Model file for the job. Use its own axes, mm. Face numbers are marked on the shaded views. A direction names the side the tool comes from. Coordinates: 2 decimals unless noted, no trailing zeros. Loops run counter-clockwise (first coordinate to the right, second up) from the corner with the lowest first, then second, coordinate; pieces in that order, holes last. Notation, with made-up numbers: M 6.5,7 L 44.5,7 A21 cw 44.5,35 Z; hole C 21,89.25 d6. An arc over 180 degrees is marked long. One line per question, with ' | ' between items. Start each with the question number.
```python
from build123d import *

# Parameters (mm, degrees)
SKETCH2_R               = 1
CUT_EXTRUDE1_DEPTH      = 5
CUT_EXTRUDE2_DEPTH      = 5
CUT_EXTRUDE3_DEPTH      = 68.470363864
CUT_EXTRUDE3_DEPTH_BACK = 68.470363864


with BuildPart() as part:
    # Sketch1 → Revolve1 (revolve)
    with BuildSketch(Plane(origin=(0, 0, 0), x_dir=(0, 0, -1), z_dir=(1, 0, 0)), mode=Mode.PRIVATE) as revolve1_sk:
        Polygon((0, 0), (1.15, 0), (1.15, 12), (5, 12), (5, 15), (14, 15), (14, 61.5), (5, 61.5), (5, 64.5), (0, 64.5), align=None)
    revolve(revolve1_sk.sketch.rotate(Axis((0, 64.5, 0), (0, -1, 0)), 180), axis=Axis((0, 64.5, 0), (0, -1, 0)))

    # Sketch2 → Cut-Extrude1 (cut)
    with BuildSketch(Plane.XZ.offset(-15)):
        with Locations(Location((-8, 0, 0), (0, 0, 270))):
            Circle(SKETCH2_R)
        with Locations(Location((8, 0, 0), (0, 0, 270))):
            Circle(SKETCH2_R)
    extrude(amount=-CUT_EXTRUDE1_DEPTH, mode=Mode.SUBTRACT)

    # Sketch3 → Cut-Extrude2 (cut)
    with BuildSketch(Plane.XZ.offset(-15)):
        with BuildLine():
            ThreePointArc((-5.070033124, 9.19482268), (-7.424621202, 7.424621202), (-9.19482268, 5.070033124))
            ThreePointArc((-9.19482268, 5.070033124), (-8.60556703, 3.03219658), (-6.567730486, 3.621452231))
            ThreePointArc((-6.567730486, 3.621452231), (-5.303300859, 5.303300859), (-3.621452231, 6.567730486))
            ThreePointArc((-3.621452231, 6.567730486), (-3.03219658, 8.60556703), (-5.070033124, 9.19482268))
        make_face()
        with BuildLine():
            ThreePointArc((6.567730486, 3.621452231), (5.303300859, 5.303300859), (3.621452231, 6.567730486))
            ThreePointArc((3.621452231, 6.567730486), (3.03219658, 8.60556703), (5.070033124, 9.19482268))
            ThreePointArc((5.070033124, 9.19482268), (7.424621202, 7.424621202), (9.19482268, 5.070033124))
            ThreePointArc((9.19482268, 5.070033124), (8.60556703, 3.03219658), (6.567730486, 3.621452231))
        make_face()
        with BuildLine():
            ThreePointArc((3.621452231, -6.567730486), (5.303300859, -5.303300859), (6.567730486, -3.621452231))
            ThreePointArc((6.567730486, -3.621452231), (8.60556703, -3.03219658), (9.19482268, -5.070033124))
            ThreePointArc((9.19482268, -5.070033124), (7.424621202, -7.424621202), (5.070033124, -9.19482268))
            ThreePointArc((5.070033124, -9.19482268), (3.03219658, -8.60556703), (3.621452231, -6.567730486))
        make_face()
        with BuildLine():
            ThreePointArc((-6.567730486, -3.621452231), (-5.303300859, -5.303300859), (-3.621452231, -6.567730486))
            ThreePointArc((-3.621452231, -6.567730486), (-3.03219658, -8.60556703), (-5.070033124, -9.19482268))
            ThreePointArc((-5.070033124, -9.19482268), (-7.424621202, -7.424621202), (-9.19482268, -5.070033124))
            ThreePointArc((-9.19482268, -5.070033124), (-8.60556703, -3.03219658), (-6.567730486, -3.621452231))
        make_face()
    extrude(amount=-CUT_EXTRUDE2_DEPTH, mode=Mode.SUBTRACT)

    # Sketch4 → Cut-Extrude3 (cut, two sides: drawn at the far end of the back side and taken through both)
    with BuildSketch(Plane(origin=(0, 0, 0), x_dir=(0, 0, -1), z_dir=(1, 0, 0)).offset(-CUT_EXTRUDE3_DEPTH_BACK)):
        with BuildLine():
            Line((-5, 56), (5, 56))
            ThreePointArc((5, 56), (7, 54), (5, 52))
            Line((5, 52), (-5, 52))
            ThreePointArc((-5, 52), (-7, 54), (-5, 56))
        make_face()
    extrude(amount=CUT_EXTRUDE3_DEPTH + CUT_EXTRUDE3_DEPTH_BACK, mode=Mode.SUBTRACT)


solid = part.part
```
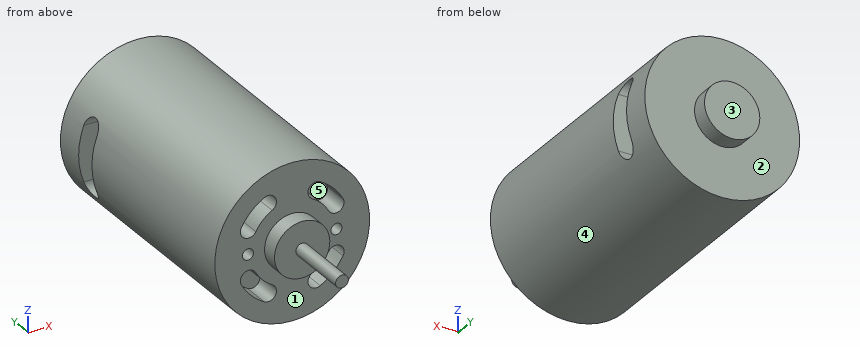
(1) Drill centre lines: line 1 (X direction, y = 17.3, z = 0); line 2 (Z direction, x = -5.5, y = 19); line 3 (Y direction, x = 7, z = -3.25). Where is each one in solid material? Low to high. Write a range as [from, to].
(2) Band-saw the part on B-B on z = 0. Write the cut outline in (x, y).
(3) Band-saw the part on A-A on x = 0. Write the cut outline in (y, z).
(4) Two-plate mould, pull along Z, no slides. Class the marked faces 3, 4 and 5: pulls with the +Z half, pulls with the -Z half, needs draft (parallel to the pull), parting line crosses it, or undercut.
(5) Band-saw the part on C-C on y = 55. Write the cut outline in (x, z).
(6) 3-axis set-ups, long thin cutter, end or side, ignore diameter. For the marked faces 1 and 2: which of +Z, -Z, +X, -X, +Y, -Y reach the whole face in a straight line?
(7) Band-saw the part on D-D on x = 10.75. Write the cut outline in (y, z), then the cut area to 3 significant figures.
(8) Pin check, flat tips, straight feed: P1, Ø1.5, axis at x = 3.5, y = 21.5, coming from the -Z side; P2, Ø3, axis at x = 3.5, z = 0, coming from the -Y side; P3, Ø5, axis at x = -6, z = -7.5, coming from the -Y side. Stop position of each tip, or through.
Computed values:
1) line 1: [-14, -9], [-7, 7], [9, 14] | line 2: [-12.87, -8.94], [-5.1, 5.1], [8.94, 12.87] | line 3: [20, 52], [56, 61.5]
2) outline: M -14,15 L -9,15 L -9,20 L -7,20 L -7,15 L -5,15 L -5,12 L -1.15,12 L -1.15,0 L 1.15,0 L 1.15,12 L 5,12 L 5,15 L 7,15 L 7,20 L 9,20 L 9,15 L 14,15 L 14,52 L -14,52 Z; M -14,56 L 14,56 L 14,61.5 L 5,61.5 L 5,64.5 L -5,64.5 L -5,61.5 L -14,61.5 Z
3) outline: M 0,-1.15 L 12,-1.15 L 12,-5 L 15,-5 L 15,-14 L 61.5,-14 L 61.5,-5 L 64.5,-5 L 64.5,5 L 61.5,5 L 61.5,14 L 15,14 L 15,5 L 12,5 L 12,1.15 L 0,1.15 Z; hole M 52,-5 A2 ccw 56,-5 L 56,5 A2 ccw 52,5 Z
4) face 3: needs draft | face 4: parting line crosses it | face 5: undercut
5) outline: M -12.28,-6.73 A14 ccw 12.28,-6.73 Z; M -12.28,6.73 L 12.28,6.73 A14 ccw Z
6) face 1: -Y | face 2: +Y
7) outline: M 15,-8.97 L 61.5,-8.97 L 61.5,8.97 L 15,8.97 Z; hole M 52,-5 A2 ccw 56,-5 L 56,5 A2 ccw 52,5 Z | area: 782 mm^2
8) P1: z = -13.73 | P2: y = 12 | P3: y = 15
